Check sheet for the modelled part. Datum: model origin and axes. Units: mm. Face numbers are marked on the shaded views. A direction names the side the tool comes from. Give positions to 0.01 mm unless a question says otherwise; leave off trailing zeros. Write each loop counter-clockwise with the first axis right and the second up, starting at its lowest first coordinate (ties: lowest second). Pieces come first, ordered by that corner, then holes. Notation, with made-up numbers: M 20.5,30 L 70.5,30 A18 ccw 70.5,65 Z; hole C 41,40.5 d7. An arc over 180 degrees is marked long. Write item = value, one per line. Start each with the question number.
1) Sectioned sample at B-B, the plane y = 15. Record the cut outline in (x, z), then the cut area to 3 significant figures.
2) Sectioned sample at A-A, the plane x = -154. Record the cut outline in (y, z), then the cut area to 3 significant figures.
3) Gauge pin test, flat ends, axial feed: pin 1 (2.5 mm diameter, centred on x = -120, z = -92, fed in from +Y); pin 2 (10 mm diameter, centred on y = 21, z = -98.5, fed in from +X). Record the tip position at first contact, or that the pin passes through.
4) Sectioned sample at D-D, the plane z = -18.5. Record the cut outline in (x, y).
5) Set-up check for the marked faces 1, 2 and 3: record each of +Z, -Z, +X, -X, +Y, -Y from which the full face is reachable in a straight line by a thin tool's end or side.
6) Sectioned sample at C-C, the plane x = 2. Record the cut outline in (y, z).
7) Draft check along Y on the marked faces 4, 5, 6 and 7. Enter one of: pulls with the +Y half, pulls with the -Y half, needs draft (parallel to the pull), parting line crosses it, or undercut.
8) Scan lines: L1, parallel to X at y = 1.95, z = -115.5; L2, parallel to Z at x = -42, y = 3; L3, parallel to X at y = 1.8, z = -99.5. Record each from-to range of solid material in increasing order.
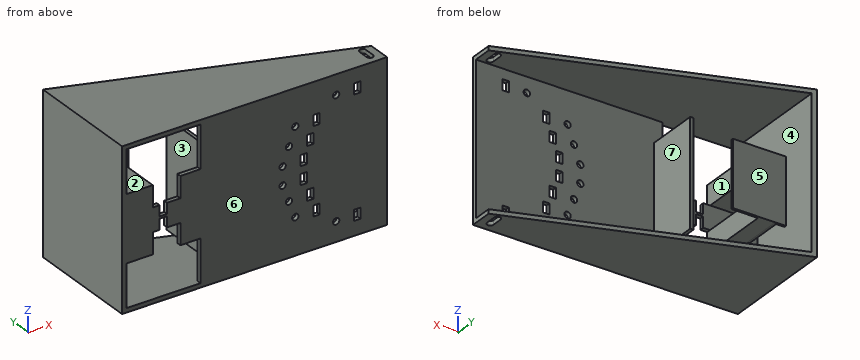
from build123d import *

# Parameters (mm, degrees)
SKETCH1_W            = 200
SKETCH1_H            = 150
SKETCH1_W_2          = 192
SKETCH1_H_2          = 142
BOSS_EXTRUDE2_DEPTH  = 4
SKETCH2_W            = 200
SKETCH2_H            = 150
SKETCH2_W_2          = 192
SKETCH2_H_2          = 142
BOSS_EXTRUDE3_DEPTH  = 80
CUT_EXTRUDE1_DEPTH   = 150
SKETCH4_R            = 3
SKETCH4_W            = 6
SKETCH4_H            = 10
CUT_EXTRUDE2_DEPTH   = 10
SKETCH5_W            = 142
SKETCH5_H            = 11.4
CUT_EXTRUDE4_DEPTH   = 10
SKETCH6_W            = 25
SKETCH6_H            = 20
BOSS_EXTRUDE4_DEPTH  = 66
SKETCH7_W            = 5
SKETCH7_H            = 37.5
CUT_EXTRUDE5_DEPTH   = 66
BOSS_EXTRUDE6_DEPTH  = 4
BOSS_EXTRUDE7_DEPTH  = 4
BOSS_EXTRUDE8_DEPTH  = 142
FILLET1_R            = 5
FILLET2_R            = 5
FILLET3_R            = 5
SKETCH15_W           = 62
SKETCH15_H           = 2
BOSS_EXTRUDE9_DEPTH  = 50
SKETCH16_W           = 6
SKETCH16_H           = 20
CUT_EXTRUDE8_DEPTH   = 50
SKETCH17_W           = 7
SKETCH17_H           = 10
CUT_EXTRUDE9_DEPTH   = 50
SKETCH18_W           = 50
SKETCH18_H           = 150
BOSS_EXTRUDE10_DEPTH = 4
SKETCH19_W           = 50
SKETCH19_H           = 4
BOSS_EXTRUDE11_DEPTH = 35
CUT_EXTRUDE10_DEPTH  = 210
SKETCH21_R           = 3
SKETCH21_W           = 6
SKETCH21_H           = 10
CUT_EXTRUDE11_DEPTH  = 30
SKETCH22_W           = 3
SKETCH22_H           = 100
BOSS_EXTRUDE12_DEPTH = 50
CUT_EXTRUDE12_DEPTH  = 150


with BuildPart() as part:
    # Sketch1 → Boss-Extrude2 (new body)
    # profile 1 of 3: a face of its own
    with BuildSketch(Plane(origin=(0, 0, 0), x_dir=(1, 0, 0), z_dir=(0, 1, 0))):
        with Locations((-100, 75)):
            Rectangle(SKETCH1_W, SKETCH1_H)
        with Locations((-100, 75)):
            Rectangle(SKETCH1_W_2, SKETCH1_H_2, mode=Mode.SUBTRACT)
    # profile 2 of 3: a face of its own
    with BuildSketch(Plane(origin=(0, 0, 0), x_dir=(1, 0, 0), z_dir=(0, 1, 0))):
        Polygon((-4, 75), (-196, 75), (-196, 44), (-171, 44), (-171, 64), (-163, 64), (-163, 74), (-159, 74), (-159, 64), (-151, 64), (-151, 44), (-126, 44), (-126, 4), (-4, 4), align=None)
    # profile 3 of 3: a face of its own
    with BuildSketch(Plane(origin=(0, 0, 0), x_dir=(1, 0, 0), z_dir=(0, 1, 0))):
        Polygon((-196, 106), (-196, 75), (-4, 75), (-4, 146), (-126, 146), (-126, 106), (-151, 106), (-151, 86), (-159, 86), (-159, 76), (-163, 76), (-163, 86), (-171, 86), (-171, 106), align=None)
    extrude(amount=BOSS_EXTRUDE2_DEPTH)

    # Sketch2 → Boss-Extrude3 (add)
    with BuildSketch(Plane(origin=(0, 4, 0), x_dir=(1, 0, 0), z_dir=(0, 1, 0))):
        with Locations((-100, 75)):
            Rectangle(SKETCH2_W, SKETCH2_H)
        with Locations((-100, 75)):
            Rectangle(SKETCH2_W_2, SKETCH2_H_2, mode=Mode.SUBTRACT)
    extrude(amount=BOSS_EXTRUDE3_DEPTH)

    # Sketch3 → Cut-Extrude1 (cut)
    with BuildSketch(Plane.XY):
        Polygon((-200, 84), (0, 14), (0, 84), align=None)
    extrude(amount=-CUT_EXTRUDE1_DEPTH, mode=Mode.SUBTRACT)

    # Sketch4 → Cut-Extrude2 (cut)
    with BuildSketch(Plane(origin=(0, 4, 0), x_dir=(1, 0, 0), z_dir=(0, 1, 0))):
        with Locations(Location((-36.5, 115.5, 0), (0, 0, 270))):
            Circle(SKETCH4_R)
        with Locations(Location((-42.5, 99.5, 0), (0, 0, 270))):
            Circle(SKETCH4_R)
        with Locations(Location((-48.5, 83.5, 0), (0, 0, 270))):
            Circle(SKETCH4_R)
        with Locations(Location((-48.5, 66.5, 0), (0, 0, 270))):
            Circle(SKETCH4_R)
        with Locations(Location((-42.5, 50.5, 0), (0, 0, 270))):
            Circle(SKETCH4_R)
        with Locations(Location((-36.5, 34.5, 0), (0, 0, 270))):
            Circle(SKETCH4_R)
        with Locations((-16.5, 34.5)):
            Rectangle(SKETCH4_W, SKETCH4_H)
        with Locations((-16.5, 115.5)):
            Rectangle(SKETCH4_W, SKETCH4_H)
        with Locations((-22.5, 99.5)):
            Rectangle(SKETCH4_W, SKETCH4_H)
        with Locations((-22.5, 50.5)):
            Rectangle(SKETCH4_W, SKETCH4_H)
        with Locations((-28.5, 66.5)):
            Rectangle(SKETCH4_W, SKETCH4_H)
        with Locations((-28.5, 83.5)):
            Rectangle(SKETCH4_W, SKETCH4_H)
    extrude(amount=-CUT_EXTRUDE2_DEPTH, mode=Mode.SUBTRACT)

    # Sketch5 → Cut-Extrude4 (cut)
    with BuildSketch(Plane(origin=(0, 0, 0), x_dir=(0, 0, -1), z_dir=(1, 0, 0))):
        with Locations((75, 9.7)):
            Rectangle(SKETCH5_W, SKETCH5_H)
    extrude(amount=-CUT_EXTRUDE4_DEPTH, mode=Mode.SUBTRACT)

    # Sketch6 → Boss-Extrude4 (add)
    with BuildSketch(Plane(origin=(0, 4, 0), x_dir=(1, 0, 0), z_dir=(0, 1, 0))):
        with Locations((-183.5, 54)):
            Rectangle(SKETCH6_W, SKETCH6_H)
        with Locations((-183.5, 96)):
            Rectangle(SKETCH6_W, SKETCH6_H)
    extrude(amount=BOSS_EXTRUDE4_DEPTH)

    # Sketch7 → Cut-Extrude5 (cut)
    with BuildSketch(Plane(origin=(0, 0, -106), x_dir=(-1, 0, 0), z_dir=(0, 0, -1))):
        with Locations((193.5, 51.25)):
            Rectangle(SKETCH7_W, SKETCH7_H)
    extrude(amount=-CUT_EXTRUDE5_DEPTH, mode=Mode.SUBTRACT)

    # Sketch12 → Boss-Extrude6 (add)
    with BuildSketch(Plane.XY):
        Polygon((-200, 84), (-200, 109), (0, 39), (0, 14), align=None)
    extrude(amount=-BOSS_EXTRUDE6_DEPTH)

    # Sketch13 → Boss-Extrude7 (add)
    with BuildSketch(Plane(origin=(0, 0, -150), x_dir=(-1, 0, 0), z_dir=(0, 0, -1))):
        Polygon((0, 14), (0, 39), (200, 109), (200, 84), align=None)
    extrude(amount=-BOSS_EXTRUDE7_DEPTH)

    # Sketch14 → Boss-Extrude8 (add)
    with BuildSketch(Plane.XY.offset(-146)):
        Polygon((-200, 84), (-200, 109), (-196, 107.6), (-196, 82.6), align=None)
    extrude(amount=BOSS_EXTRUDE8_DEPTH)

    # Fillet1
    fillet1_edges = [part.edges().sort_by_distance(p)[0] for p in [
        (-191, 51.25, -106),
    ]]
    fillet(fillet1_edges, radius=FILLET1_R)

    # Fillet2
    fillet2_edges = [part.edges().sort_by_distance(p)[0] for p in [
        (-191, 51.25, -86),
    ]]
    fillet(fillet2_edges, radius=FILLET2_R)

    # Fillet3
    fillet3_edges = [part.edges().sort_by_distance(p)[0] for p in [
        (-191, 51.25, -44),
        (-191, 51.25, -64),
    ]]
    fillet(fillet3_edges, radius=FILLET3_R)

    # Sketch15 → Boss-Extrude9 (add)
    with BuildSketch(Plane(origin=(-196, 0, 0), x_dir=(0, 0, -1), z_dir=(1, 0, 0))):
        with Locations((75, 71)):
            Rectangle(SKETCH15_W, SKETCH15_H)
    extrude(amount=BOSS_EXTRUDE9_DEPTH)

    # Sketch16 → Cut-Extrude8 (cut)
    with BuildSketch(Plane(origin=(0, 4, 0), x_dir=(1, 0, 0), z_dir=(0, 1, 0))):
        with Locations((-148, 96)):
            Rectangle(SKETCH16_W, SKETCH16_H)
        with Locations((-148, 54)):
            Rectangle(SKETCH16_W, SKETCH16_H)
    extrude(amount=-CUT_EXTRUDE8_DEPTH, mode=Mode.SUBTRACT)

    # Sketch17 → Cut-Extrude9 (cut)
    with BuildSketch(Plane(origin=(0, 4, 0), x_dir=(1, 0, 0), z_dir=(0, 1, 0))):
        with Locations((-161, 69)):
            Rectangle(SKETCH17_W, SKETCH17_H)
        with Locations((-161, 81)):
            Rectangle(SKETCH17_W, SKETCH17_H)
    extrude(amount=-CUT_EXTRUDE9_DEPTH, mode=Mode.SUBTRACT)

    # Sketch18 → Boss-Extrude10 (add)
    with BuildSketch(Plane.XZ):
        with Locations((25, -75)):
            Rectangle(SKETCH18_W, SKETCH18_H)
    extrude(amount=-BOSS_EXTRUDE10_DEPTH)

    # Sketch19 → Boss-Extrude11 (add)
    with BuildSketch(Plane(origin=(0, 4, 0), x_dir=(1, 0, 0), z_dir=(0, 1, 0))):
        with Locations((25, 148)):
            Rectangle(SKETCH19_W, SKETCH19_H)
        with Locations((25, 2)):
            Rectangle(SKETCH19_W, SKETCH19_H)
    extrude(amount=BOSS_EXTRUDE11_DEPTH)

    # Sketch20 → Cut-Extrude10 (cut)
    with BuildSketch(Plane.XY):
        Polygon((0, 39), (50, 21.5), (50, 39), align=None)
    extrude(amount=-CUT_EXTRUDE10_DEPTH, mode=Mode.SUBTRACT)

    # Sketch21 → Cut-Extrude11 (cut)
    with BuildSketch(Plane(origin=(0, 4, 0), x_dir=(1, 0, 0), z_dir=(0, 1, 0))):
        with Locations(Location((2, 131.5, 0), (0, 0, 270))):
            Circle(SKETCH21_R)
        with Locations(Location((2, 18.5, 0), (0, 0, 270))):
            Circle(SKETCH21_R)
        with Locations((22, 18.5)):
            Rectangle(SKETCH21_W, SKETCH21_H)
        with Locations((22, 131.5)):
            Rectangle(SKETCH21_W, SKETCH21_H)
    extrude(amount=-CUT_EXTRUDE11_DEPTH, mode=Mode.SUBTRACT)

    # Sketch22 → Boss-Extrude12 (add)
    with BuildSketch(Plane(origin=(0, 4, 0), x_dir=(1, 0, 0), z_dir=(0, 1, 0))):
        with Locations((-119.5, 75)):
            Rectangle(SKETCH22_W, SKETCH22_H)
    extrude(amount=BOSS_EXTRUDE12_DEPTH)

    # Sketch23 → Cut-Extrude12 (cut)
    with BuildSketch(Plane(origin=(0, 0, -150), x_dir=(-1, 0, 0), z_dir=(0, 0, -1))):
        with BuildLine():
            Line((-43, 9), (-43, 19))
            ThreePointArc((-43, 19), (-40, 22), (-37, 19))
            Line((-37, 19), (-37, 9))
            ThreePointArc((-37, 9), (-40, 6), (-43, 9))
        make_face()
    extrude(amount=-CUT_EXTRUDE12_DEPTH, mode=Mode.SUBTRACT)


solid = part.part
Data:
q1.outline = M -200,-150 L 37,-150 L 37,-146 L -196,-146 L -196,-106 L -171,-106 L -171,-86 L -196,-86 L -196,-64 L -171,-64 L -171,-44 L -196,-44 L -196,-4 L 37,-4 L 37,0 L -200,0 Z; M -121,-125 L -118,-125 L -118,-25 L -121,-25 Z; M 43,-150 L 50,-150 L 50,-146 L 43,-146 Z; M 43,-4 L 50,-4 L 50,0 L 43,0 Z
q1.area = 3,820 mm2
q2.outline = M 0,-150 L 92.9,-150 L 92.9,-146 L 0,-146 Z; M 0,-86 L 4,-86 L 4,-64 L 0,-64 Z; M 0,-4 L 92.9,-4 L 92.9,0 L 0,0 Z; M 70,-106 L 72,-106 L 72,-44 L 70,-44 Z
q2.area = 955 mm2
q3.pin_1 = 54
q3.pin_2 = -118
q4.outline = M -200,0 L -196,0 L -196,107.6 L -200,109 Z; M -126,0 L -1,0 L -1,4 L -126,4 Z; M 5,0 L 19,0 L 19,4 L 5,4 Z; M 25,0 L 50,0 L 50,4 L 25,4 Z
q5.face_1 = -Y
q5.face_2 = +Y, -Y
q5.face_3 = +Y
q6.outline = M 0,-150 L 38.3,-150 L 38.3,-146 L 4,-146 L 4,-134.5 L 0,-134.5 Z; M 0,-128.5 L 4,-128.5 L 4,-21.5 L 0,-21.5 Z; M 0,-15.5 L 4,-15.5 L 4,-4 L 38.3,-4 L 38.3,0 L 0,0 Z
q7.face_4 = undercut
q7.face_5 = pulls with the +Y half
q7.face_6 = pulls with the -Y half
q7.face_7 = needs draft
q8.L1 = -200 to -196, -126 to -39.5, -33.5 to -19.5, -13.5 to 50
q8.L2 = -150 to -102.46, -96.54 to -53.46, -47.54 to 0
q8.L3 = -200 to -171, -145 to -45.5, -39.5 to -25.5, -19.5 to 50
